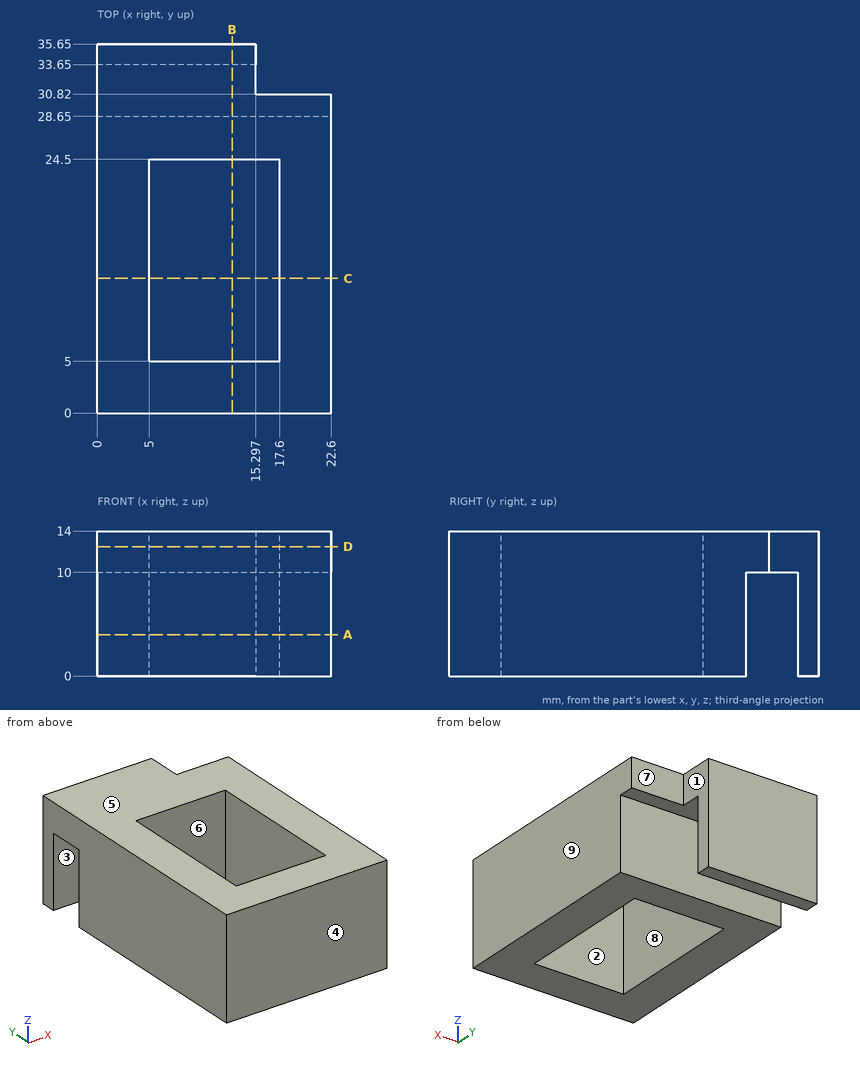
Input: dimensioned drawing with shaded views. Units: mm. Origin: part minimum x, y, z. A direction names the side the tool comes from. Give positions to 0.01 mm unless a question says otherwise; leave off trailing zeros. Write each loop counter-clockwise with the first axis right and the second up, starting at its lowest first coordinate (ties: lowest second). Pieces come first, ordered by that corner, then holes. Notation, with made-up numbers: (74, -17.5) - (78, -17.5) arc R23 ccw to (78, -7.5) - close; hole circle Ø7 at (-32, 45). An arc over 180 degrees is marked (long way). Write item = value, one per line. Start each with the question number.
1) Pin query (flat end, axial travel): pin 1 (2.5 mm diameter, centred on y = 33, z = 5.5, fed in from +X); pin 2 (1.5 mm diameter, centred on x = 10, y = 30, fed in from -Z); pin 3 (2 mm diameter, centred on x = 19, z = 12.5, fed in from +Y). Return the tip coordinate at first contact, or that it passes through.
2) Cut plane C-C (y = 13). Return loops of the section in (x, z).
3) Material intervals for L1, parallel to Y at x = 7.25, z = 4; L2, parallel to X at y = 16.5, z = 13.5; L3, parallel to Y at x = 17, z = 13, sorted ascending. Write a range as [from, to].
4) Cut plane D-D (z = 12.5). Return loops of the section in (x, y).
5) Draft query along Y for the marked faces 6, 7, 8 and 9. Return one class per face: pulls with the +Y half, pulls with the -Y half, needs draft (parallel to the pull), parting line crosses it, or undercut.
6) Reachability of the marked faces 1, 2, 3, 4 and 5 from +Z, -Z, +X, -X, +Y, -Y: full face, straight path, thin tool, end or side. Return the list, or none.
7) Cut plane A-A (z = 4). Return loops of the section in (x, y).
8) Cut plane B-B (x = 13). Return loops of the section in (y, z).
Answers follow:
q1.pin_1 = 15.3
q1.pin_2 = 10
q1.pin_3 = 30.82
q2.outline = (0, 0) - (5, 0) - (5, 14) - (0, 14) - close; (17.6, 0) - (22.6, 0) - (22.6, 14) - (17.6, 14) - close
q3.L1 = [0, 5], [24.5, 28.65], [33.65, 35.65]
q3.L2 = [0, 5], [17.6, 22.6]
q3.L3 = [0, 5], [24.5, 30.82]
q4.outline = (0, 0) - (22.6, 0) - (22.6, 30.82) - (15.3, 30.82) - (15.3, 35.65) - (0, 35.65) - close; hole (5, 5) - (17.6, 5) - (17.6, 24.5) - (5, 24.5) - close
q5.face_6 = undercut
q5.face_7 = pulls with the +Y half
q5.face_8 = undercut
q5.face_9 = needs draft
q6.face_1 = +Z, -Z, +X, +Y
q6.face_2 = +Z, -Z
q6.face_3 = -Z, +X, -X
q6.face_4 = +Z, -Z, +X, -X, -Y
q6.face_5 = +Z, +X, -X, +Y, -Y
q7.outline = (0, 0) - (22.6, 0) - (22.6, 28.65) - (0, 28.65) - close; (0, 33.65) - (15.3, 33.65) - (15.3, 35.65) - (0, 35.65) - close; hole (5, 5) - (17.6, 5) - (17.6, 24.5) - (5, 24.5) - close
q8.outline = (0, 0) - (5, 0) - (5, 14) - (0, 14) - close; (24.5, 0) - (28.65, 0) - (28.65, 10) - (33.65, 10) - (33.65, 0) - (35.65, 0) - (35.65, 14) - (24.5, 14) - close
